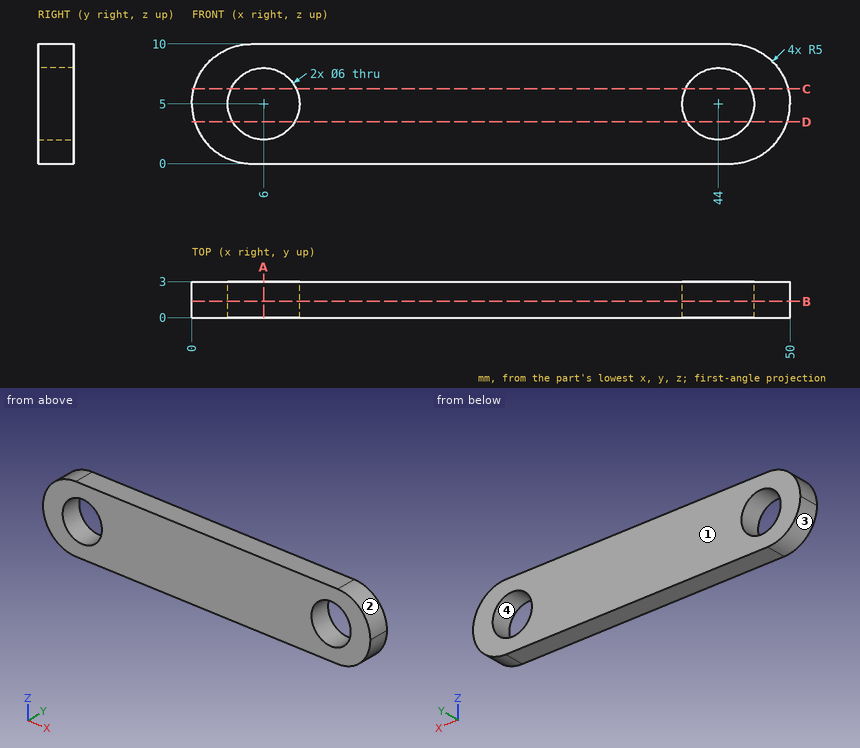
Design review of the part shown in the three views and the two pictorial views. Dimensions are in mm from the part's minimum x, y and z. Round coordinates to 2 decimals unless told otherwise and drop trailing zeros. Write each loop counter-clockwise with the first axis right and the second up, starting at its lowest first coordinate (ties: lowest second). Pieces come first, ordered by that corner, then holes.
1) For line 1 along X through (y, z) = (1.35, 5); line 2 along X through (y, z) = (1.95, 3.75); line 3 along X through (y, z) = (2.4, 1.75), list the stretches that pass through material, from the lowest coordinate up.
Answer below:
line 1: x = 0 to 3, 9 to 41, 47 to 50
line 2: x = 0.16 to 3.27, 8.73 to 41.27, 46.73 to 49.84
line 3: x = 1.2 to 48.8
2) Mouldability with a two-part tool opening along Z and no side actions: class the marked faces 1, 2, 3 and 4 as +Z half, -Z half, draft (parallel to the pull), parting line (faces both ways), or undercut.
Answer below:
face 1: draft
face 2: +Z half
face 3: -Z half
face 4: undercut
3) Take a section at D-D on z = 3.5. Give the boundary of the cut face in (x, y).
Answer below:
outline: (0.23, 0) - (3.4, 0) - (3.4, 3) - (0.23, 3) - close; (8.6, 0) - (41.4, 0) - (41.4, 3) - (8.6, 3) - close; (46.6, 0) - (49.77, 0) - (49.77, 3) - (46.6, 3) - close
4) Take a section at B-B on y = 1.35. State how many separate pieces and enclosed holes the cut face has, then the cut area to 3 significant figures.
Answer below:
separate pieces: 1
enclosed holes: 2
area: 422 mm2
5) Take a section at C-C on z = 6.25. Give the boundary of the cut face in (x, y).
Answer below:
outline: (0.16, 0) - (3.27, 0) - (3.27, 3) - (0.16, 3) - close; (8.73, 0) - (41.27, 0) - (41.27, 3) - (8.73, 3) - close; (46.73, 0) - (49.84, 0) - (49.84, 3) - (46.73, 3) - close
6) Take a section at A-A on x = 6. Give the boundary of the cut face in (y, z), then the cut area to 3 significant figures.
Answer below:
outline: (0, 0) - (3, 0) - (3, 2) - (0, 2) - close; (0, 8) - (3, 8) - (3, 10) - (0, 10) - close
area: 12.0 mm2
